Build history of the part. All positions in model axes, mm. Face numbers are marked on the shaded views. A direction names the side the tool comes from. Round coordinates to 2 decimals unless told otherwise and drop trailing zeros. Order: outer loops, then holes, each group sorted by start corner. A loop starts at its lowest first (then second) coordinate and runs counter-clockwise, first axis right, second up. Notation, with made-up numbers: (-0.75, 6.5) -> (20.25, 6.5) arc R28 ccw to (20.25, 32.5) -> close; hole circle Ø7 at (37, -39). An arc over 180 degrees is marked (long way). Write item = value, one per line.
from build123d import *

# Parameters (mm, degrees)
SCHIZZO1_W                   = 13
SCHIZZO1_H                   = 2.5
ESTRUSIONE_ESTRUSIONE1_DEPTH = 3
ESTRUSIONE_ESTRUSIONE2_DEPTH = 6
SCHIZZO3_R                   = 1
TAGLIO_ESTRUSIONE1_DEPTH     = 7
TAGLIO_ESTRUSIONE2_DEPTH     = 0.5
SMUSSO1_SIZE                 = 0.5
ESTRUSIONE_ESTRUSIONE3_DEPTH = 0.4
RIPETIZIONE_A_L1_COUNT       = 2
RIPETIZIONE_A_L1_PITCH       = 5.2
RIPETIZIONE_A_L1_COL_COUNT   = 2
RIPETIZIONE_A_L1_COL_PITCH   = 5.2


with BuildPart() as part:
    # Schizzo1 → Estrusione-Estrusione1 (new body, symmetric)
    with BuildSketch(Plane.XY):
        Rectangle(SCHIZZO1_W, SCHIZZO1_H)
    extrude(amount=ESTRUSIONE_ESTRUSIONE1_DEPTH, both=True)

    # Schizzo2 → Estrusione-Estrusione2 (add)
    with BuildSketch(Plane.XY.offset(3)):
        Polygon((-4.8, -1.25), (-4.3, -1.75), (-2.3, -1.75), (-1.8, -1.25), (1.8, -1.25), (2.3, -1.75), (4.3, -1.75), (4.8, -1.25), (4.8, -0.938044121), (-4.8, -0.938044121), align=None)
    extrude(amount=-ESTRUSIONE_ESTRUSIONE2_DEPTH)

    # Schizzo3 → Taglio-Estrusione1 (cut, through all)
    with BuildSketch(Plane.XY.offset(3)):
        with Locations((-3.25, -0.25)):
            Circle(SCHIZZO3_R)
        with Locations((3.25, -0.25)):
            Circle(SCHIZZO3_R)
    extrude(amount=-TAGLIO_ESTRUSIONE1_DEPTH, mode=Mode.SUBTRACT)

    # Schizzo4 → Taglio-Estrusione2 (cut)
    with BuildSketch(Plane.XY.offset(3)):
        Polygon((-1.8, 1.25), (-0.501117074, 1.25), (-0.501117074, 0.25), (0.498882926, 0.25), (0.498882926, 1.25), (1.8, 1.25), (1.8, -0.75), (-1.8, -0.75), align=None)
    taglio_estrusione2 = extrude(amount=-TAGLIO_ESTRUSIONE2_DEPTH, mode=Mode.SUBTRACT)

    # Specchia2: Taglio-Estrusione2 across plane
    add(taglio_estrusione2.mirror(Plane.XY), mode=Mode.SUBTRACT)

    # Smusso1
    smusso1_edges = [part.edges().sort_by_distance(p)[0] for p in [
        (-0.001117074, 1.25, 3),
        (-0.001117074, 1.25, -3),
    ]]
    chamfer(smusso1_edges, length=SMUSSO1_SIZE)

    # Schizzo5 → Estrusione-Estrusione3 (add, symmetric)
    with BuildSketch(Plane(origin=(0, 0, 0), x_dir=(0, 0, -1), z_dir=(1, 0, 0))):
        with BuildLine():
            Line((-0.3, -1.25), (-0.3, -2.85))
            ThreePointArc((-0.3, -2.85), (-0.007106781, -3.557106781), (0.7, -3.85))
            Line((0.7, -3.85), (5, -3.85))
            Line((5, -3.85), (5, -3.25))
            Line((5, -3.25), (0.7, -3.25))
            ThreePointArc((0.7, -3.25), (0.417157288, -3.132842712), (0.3, -2.85))
            Line((0.3, -2.85), (0.3, -1.25))
            Line((0.3, -1.25), (-0.3, -1.25))
        make_face()
    estrusione_estrusione3 = extrude(amount=ESTRUSIONE_ESTRUSIONE3_DEPTH, both=True)

    # Ripetizione a L1: Estrusione-Estrusione3 ×2
    with Locations(*[(-i * RIPETIZIONE_A_L1_PITCH, 0, 0) for i in range(1, RIPETIZIONE_A_L1_COUNT)]):
        add(estrusione_estrusione3)

    # Ripetizione a L1 col: Estrusione-Estrusione3 ×2
    with Locations(*[(i * RIPETIZIONE_A_L1_COL_PITCH, 0, 0) for i in range(1, RIPETIZIONE_A_L1_COL_COUNT)]):
        add(estrusione_estrusione3)


solid = part.part
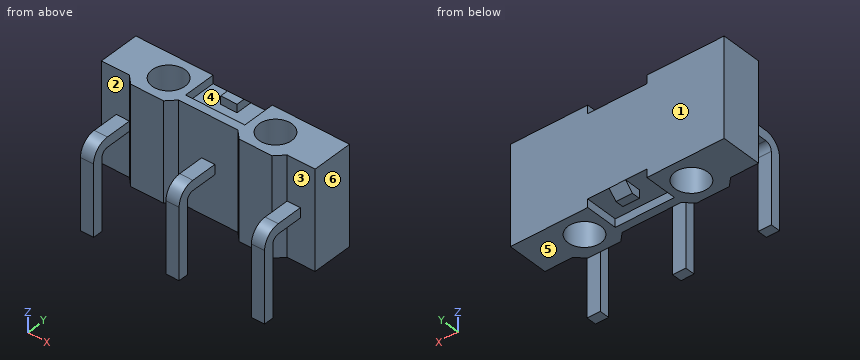
Q1. Which spindle directions (+Z, -Z, +X, -X, +Y, -Y) get a long thin tool onto all of the face, cutting with end or side? Do the marked faces 1, 2 and 3. Say none if no direction does.
Check values:
face_1 = +Z, -Z, +X, -X, +Y
face_2 = -X
face_3 = +X
Q2. Cut at B-B, the plane y = -0.25. List the corners of the cut face in (x, z), and give its area (3 significant figures).
Check values:
outline = (-6.5, -3) -> (-4.25, -3) -> (-4.25, 3) -> (-6.5, 3) -> close; (-2.25, -3) -> (-1.8, -3) -> (-1.8, -2.5) -> (1.8, -2.5) -> (1.8, -3) -> (2.25, -3) -> (2.25, 3) -> (1.8, 3) -> (1.8, 2.5) -> (-1.8, 2.5) -> (-1.8, 3) -> (-2.25, 3) -> close; (4.25, -3) -> (6.5, -3) -> (6.5, 3) -> (4.25, 3) -> close
area = 50.4 mm²
Q3. Cut at A-A, the plane z = -1.5. List the corners of the cut face in (x, y), and give its area (3 significant figures).
Check values:
outline = (-6.5, -1.25) -> (-4.8, -1.25) -> (-4.3, -1.75) -> (-2.3, -1.75) -> (-1.8, -1.25) -> (1.8, -1.25) -> (2.3, -1.75) -> (4.3, -1.75) -> (4.8, -1.25) -> (6.5, -1.25) -> (6.5, 1.25) -> (-6.5, 1.25) -> close; (-5.6, -3.85) -> (-4.8, -3.85) -> (-4.8, -3.25) -> (-5.6, -3.25) -> close; (-0.4, -3.85) -> (0.4, -3.85) -> (0.4, -3.25) -> (-0.4, -3.25) -> close; (4.8, -3.85) -> (5.6, -3.85) -> (5.6, -3.25) -> (4.8, -3.25) -> close; hole circle Ø2 at (-3.25, -0.25); hole circle Ø2 at (3.25, -0.25)
area = 30.2 mm²
Q4. Flat gauge pins, fed straight in: pin 1 (1.3 mm diameter, centred on y = -3, z = -1, fed in from +X); pin 2 (1.9 mm diameter, centred on x = -6, z = 0.5, fed in from -Y); pin 3 (1 mm diameter, centred on x = 3, z = -2.5, fed in from -Y). Where does each tip first touch, or does it go through?
Check values:
pin_1 = 5.6
pin_2 = -3.79
pin_3 = -1.75
Q5. Probe probe 1 along X at (y, z) = (-0.3, 0); probe 2 along Y at (x, z) = (3.25, 1.35); probe 3 along X at (y, z) = (-2.55, 0). List the from-to ranges inside material, lowest first.
Check values:
probe_1 = -6.5 to -4.25, -2.25 to 2.25, 4.25 to 6.5
probe_2 = -1.75 to -1.25, 0.75 to 1.25
probe_3 = -5.6 to -4.8, -0.4 to 0.4, 4.8 to 5.6
Q6. Cut at C-C, the plane x = -3.25. List the corners of the cut face in (y, z).
Check values:
outline = (-1.75, -3) -> (-1.25, -3) -> (-1.25, 3) -> (-1.75, 3) -> close; (0.75, -3) -> (1.25, -3) -> (1.25, 3) -> (0.75, 3) -> close
Q7. Mould opens along X. For the marked faces 4, 5 and 6 say: released by +X, released by -X, zero draft, split by the parting line, or undercut.
Check values:
face_4 = undercut
face_5 = zero draft
face_6 = released by +X
Q8. Cut at D-D, the plane x = -5. List the corners of the cut face in (y, z).
Check values:
outline = (-3.85, -5) -> (-3.25, -5) -> (-3.25, -0.7) arc R0.4 cw to (-2.85, -0.3) -> (-1.25, -0.3) -> (-1.25, -3) -> (1.25, -3) -> (1.25, 3) -> (-1.25, 3) -> (-1.25, 0.3) -> (-2.85, 0.3) arc R1 ccw to (-3.85, -0.7) -> close
